Check sheet for the modelled part. Datum: model origin and axes. Units: mm. Give positions to 0.01 mm unless a question says otherwise; leave off trailing zeros. Loops run counter-clockwise (first coordinate to the right, second up) from the corner with the lowest first, then second, coordinate; pieces in that order, holes last. Notation, with made-up numbers: (-13, -0.75) - (29, -0.75) arc R27 cw to (29, 22.25) - close; hole circle Ø5 at (73, -12.5). An arc over 180 degrees is marked (long way). Answer in a Markdown table with one row per item. Add a question column.
(1) Sectioned sample at B-B on y = 0. Enter the section's corners in (x, z) (3 decimals).
(2) Sectioned sample at D-D on x = 46.5. Enter the section's corners in (y, z) (3 decimals), then the cut area to 3 significant figures.
(3) Sectioned sample at A-A on x = -10. Enter the section's corners in (y, z) (3 decimals), then the cut area to 3 significant figures.
(4) Draft check along Y on faces 1 (the face through (-2, 2, 3.175)), 2 (the face through (-97.804, -0.363, 1.61)). Enter one of: released by +Y, released by -Y, zero draft, split by the parting line, or undercut.
(5) Thickness scan on L1, parallel to X at y = -19, z = 2.8; L2, parallel to Y at x = 10, z = 2.75 (3 decimals); L3, parallel to X at y = 3, z = 0.3 (3 decimals). Record the ranges inside material, lowest first.
(6) Sectioned sample at C-C on z = 0.5. State how many separate pieces and enclosed holes the cut face has, then the cut area to 3 significant figures.
(7) Go/stop test with flat-tipped pins: P1, Ø1, axis at y = 3, z = 1, coming from the -X side; P2, Ø1, axis at x = 100.5, z = 1, coming from the +Y side; P3, Ø1.6, axis at y = -6.5, z = 2.5, coming from the -X side. Record where each tip stops, or that it passes through.
from build123d import *

# Parameters (mm, degrees)
SKETCH1_W           = 228.6
SKETCH1_H           = 50.8
BOSS_EXTRUDE1_DEPTH = 3.175
SKETCH2_W           = 30
SKETCH2_H           = 3.175
BOSS_EXTRUDE2_DEPTH = 3.175
SKETCH3_R           = 16.5
CUT_EXTRUDE1_DEPTH  = 4.175
SKETCH4_W           = 3.175
SKETCH4_H           = 30
SKETCH4_H_2         = 15
CUT_EXTRUDE2_DEPTH  = 10
SKETCH5_W           = 31
SKETCH5_H           = 3.175
CUT_EXTRUDE3_DEPTH  = 10
FILLET1_R           = 1


with BuildPart() as part:
    # Sketch1 → Boss-Extrude1 (new body)
    with BuildSketch(Plane.XY):
        Rectangle(SKETCH1_W, SKETCH1_H)
    extrude(amount=BOSS_EXTRUDE1_DEPTH)

    # Sketch2 → Boss-Extrude2 (add)
    with BuildSketch(Plane(origin=(0, 25.4, 0), x_dir=(1, 0, 0), z_dir=(0, 1, 0))):
        with Locations((69.3, -1.5875)):
            Rectangle(SKETCH2_W, SKETCH2_H)
        with Locations((9.3, -1.5875)):
            Rectangle(SKETCH2_W, SKETCH2_H)
        with Locations((-50.7, -1.5875)):
            Rectangle(SKETCH2_W, SKETCH2_H)
    extrude(amount=BOSS_EXTRUDE2_DEPTH)

    # Sketch3 → Cut-Extrude1 (cut, through all)
    with BuildSketch(Plane.XY.offset(3.175)):
        with Locations((-114.3, 0)):
            Circle(SKETCH3_R)
    extrude(amount=-CUT_EXTRUDE1_DEPTH, mode=Mode.SUBTRACT)

    # Sketch4 → Cut-Extrude2 (cut)
    with BuildSketch(Plane.XY.offset(3.175)):
        with Locations((106.3625, 0)):
            Rectangle(SKETCH4_W, SKETCH4_H)
        with Locations((38.0375, 0.9)):
            Rectangle(SKETCH4_W, SKETCH4_H_2)
        with Locations((-37.1875, 0.9)):
            Rectangle(SKETCH4_W, SKETCH4_H_2)
    extrude(amount=-CUT_EXTRUDE2_DEPTH, mode=Mode.SUBTRACT)

    # Sketch5 → Cut-Extrude3 (cut)
    with BuildSketch(Plane.XY.offset(3.175)):
        with Locations((-3.1, -19.8125)):
            Rectangle(SKETCH5_W, SKETCH5_H)
    extrude(amount=-CUT_EXTRUDE3_DEPTH, mode=Mode.SUBTRACT)

    # Fillet1
    fillet1_edges = [part.edges().sort_by_distance(p)[0] for p in [
        (-38.775, -6.6, 1.5875),
        (-38.775, 8.4, 1.5875),
        (-35.6, 8.4, 1.5875),
        (-35.6, -6.6, 1.5875),
        (104.775, -15, 1.5875),
        (104.775, 15, 1.5875),
        (107.95, 15, 1.5875),
        (107.95, -15, 1.5875),
        (39.625, 8.4, 1.5875),
        (39.625, -6.6, 1.5875),
        (36.45, -6.6, 1.5875),
        (36.45, 8.4, 1.5875),
        (12.4, -18.225, 1.5875),
        (12.4, -21.4, 1.5875),
        (-18.6, -21.4, 1.5875),
        (-18.6, -18.225, 1.5875),
        (84.3, 28.575, 1.5875),
        (54.3, 28.575, 1.5875),
        (-5.7, 28.575, 1.5875),
        (24.3, 28.575, 1.5875),
        (-65.7, 28.575, 1.5875),
        (-35.7, 28.575, 1.5875),
    ]]
    fillet(fillet1_edges, radius=FILLET1_R)


solid = part.part
Reply:
| question | item | result |
|---|---|---|
| 1 | outline | (-97.8, 0) - (-38.775, 0) - (-38.775, 3.175) - (-97.8, 3.175) - close; (-35.6, 0) - (36.45, 0) - (36.45, 3.175) - (-35.6, 3.175) - close; (39.625, 0) - (104.775, 0) - (104.775, 3.175) - (39.625, 3.175) - close; (107.95, 0) - (114.3, 0) - (114.3, 3.175) - (107.95, 3.175) - close |
| 2 | outline | (-25.4, 0) - (25.4, 0) - (25.4, 3.175) - (-25.4, 3.175) - close |
| 2 | area | 161 mm^2 |
| 3 | outline | (-25.4, 0) - (-21.4, 0) - (-21.4, 3.175) - (-25.4, 3.175) - close; (-18.225, 0) - (25.4, 0) - (25.4, 3.175) - (-18.225, 3.175) - close |
| 3 | area | 151 mm^2 |
| 4 | face 1 | zero draft |
| 4 | face 2 | undercut |
| 5 | L1 | -114.3 to -18.57, 12.37 to 114.3 |
| 5 | L2 | -25.4 to -21.4, -18.225 to 28.575 |
| 5 | L3 | -98.075 to -38.775, -35.6 to 36.45, 39.625 to 104.775, 107.95 to 114.3 |
| 6 | separate pieces | 1 |
| 6 | enclosed holes | 4 |
| 6 | area | 11,200 mm^2 |
| 7 | P1 | x = -98.18 |
| 7 | P2 | y = 25.4 |
| 7 | P3 | x = -99.5 |
